Here's how the part is built. I have some questions about the finished solid (model axes, mm). Coordinates: 2 decimals unless noted, no trailing zeros. Loops run counter-clockwise (first coordinate to the right, second up) from the corner with the lowest first, then second, coordinate; pieces in that order, holes last. Notation, with made-up numbers: (28.25, 17.25) - (73.25, 17.25) arc R29 ccw to (73.25, 49.25) - close; hole circle Ø11 at (71, 48). An arc over 180 degrees is marked (long way). Use a Markdown table: item, result.
```python
from build123d import *

# Parameters (mm, degrees)
F0_R     = 25.4
F1_DEPTH = 50.8
F3_ANGLE = -180


with BuildPart() as f1:
    # F0 (on Top) → F1 (new body)
    with BuildSketch(Plane.XY):
        Circle(F0_R)
    extrude(amount=F1_DEPTH)

    # F2 (on Front) → F3 (revolve, cut)
    with BuildSketch(Plane.XZ):
        with BuildLine():
            Line((0, 31.75), (0, 69.849997))
            ThreePointArc((0, 69.849997), (-19.050003, 50.799999), (0, 31.75))
        make_face()
    revolve(axis=Axis((0, 0, 50.799999), (0, 0, -1)), revolution_arc=F3_ANGLE, mode=Mode.SUBTRACT)

    # F2 (on Front) → F4 (revolve, cut)
    with BuildSketch(Plane.XZ):
        with BuildLine():
            Line((0, 31.75), (0, 69.849997))
            ThreePointArc((0, 69.849997), (-19.050003, 50.799999), (0, 31.75))
        make_face()
    revolve(axis=Axis((0, 0, 0), (0, 0, -1)), mode=Mode.SUBTRACT)


solid = f1.part
```
Q1. Please list where these lines run through material, in increasing order: L1, parallel to X at y = -15, z = 41; L2, parallel to Y at x = 0, z = 6; L3, parallel to Y at x = 6, z = 47.5. Write a range as from..to.
Check values:
| item | result |
|---|---|
| L1 | -20.5..-6.47, 6.47..20.5 |
| L2 | -25.4..25.4 |
| L3 | -24.68..-17.78, 17.78..24.68 |
Q2. Will these pins go through, and if not, where does the flat tip stop? P1, Ø5, axis at x = 0.5, z = 21, coming from the +Y side; P2, Ø3, axis at y = -17.5, z = 27.5, coming from the -X side; P3, Ø8, axis at x = 3, z = 42, coming from the -Y side.
Check values:
| item | result |
|---|---|
| P1 | y = 25.4 |
| P2 | x = -19.73 |
| P3 | y = -25.4 |
Q3. I want a section at A-A, the plane z = 30.5. Write out the boundary of the cut face in (x, y), then the cut area to 3 significant figures.
Check values:
| item | result |
|---|---|
| outline | circle Ø50.8 at (0, 0) |
| area | 2,030 mm^2 |
Q4. I want a section at B-B, the plane y = 22. Write out the boundary of the cut face in (x, z).
Check values:
| item | result |
|---|---|
| outline | (-12.69, 0) - (12.69, 0) - (12.69, 50.8) - (-12.69, 50.8) - close |
Q5. If we mould it in two halves opening along X, with no side actions, what happens to faces 1 (the face through (-5.506, -24.796, 25.044)), 2 (the face through (0, 0, 0))? For each: pulls with the +X half, pulls with the -X half, needs draft (parallel to the pull), parting line crosses it, or undercut.
Check values:
| item | result |
|---|---|
| face 1 | parting line crosses it |
| face 2 | needs draft |
